Build history of the part. All positions in model axes, mm. A direction names the side the tool comes from. Round coordinates to 2 decimals unless told otherwise and drop trailing zeros. Order: outer loops, then holes, each group sorted by start corner. A loop starts at its lowest first (then second) coordinate and runs counter-clockwise, first axis right, second up. Notation, with made-up numbers: M 1,42.5 L 57,42.5 A17 ccw 57,49.5 Z; hole C 39,78 d6. An arc over 180 degrees is marked long. Use CSV: the item, a comma, the result in double quotes.
Autodesk Fusion 360 part; units mm, degrees
sketch "Sketch1" plane through (0, 0, 0) normal (0, 0, 1) x (1, 0, 0)
  line L0 (22, 1.5) -> (22, -1.5)
  line L1 (-22, -1.5) -> (-22, 1.5)
  circle A0 centre (-17.5, 0) radius 2.05
  circle A1 centre (17.5, 0) radius 2.05
  line L2 (-20, 3.5) -> (-13.5554, 3.5)
  line L3 (13.5554, 3.5) -> (20, 3.5)
  line L4 (20, -3.5) -> (13.5554, -3.5)
  line L5 (-13.5554, -3.5) -> (-20, -3.5)
  arc A2 (2.9858, -13.6779) -> (13.5554, -3.5) centre (0, 0) ccw
  arc A3 (22, 1.5) -> (20, 3.5) centre (20, 1.5) ccw
  arc A4 (20, -3.5) -> (22, -1.5) centre (20, -1.5) ccw
  arc A5 (-20, 3.5) -> (-22, 1.5) centre (-20, 1.5) ccw
  arc A6 (-22, -1.5) -> (-20, -3.5) centre (-20, -1.5) ccw
  circle A7 centre (0, 8) radius 4.55
  circle A8 centre (0, 8) radius 2.5
  spline S0 degree 5 poles (-13.5554, 3.5) (-13.4403, 3.6899) (-13.2044, 4.0607) (-12.8333, 4.5904) (-12.3036, 5.2425) (-11.5792, 5.9613) (-10.7872, 6.5756) (-9.9224, 7.0772) (-8.9826, 7.4626) (-7.9714, 7.7375) (-6.8944, 7.9106) (-5.9846, 7.9745) (-5.2769, 7.9832) (-4.794, 7.9718) (-4.5498, 7.9619) knots 0 0 0 0 0 0 0.1 0.2 0.3 0.4 0.5 0.6 0.7 0.8 0.9 1 1 1 1 1 1
  spline S1 degree 5 poles (13.5554, 3.5) (13.4982, 3.7035) (13.3727, 4.1002) (13.1508, 4.664) (12.7869, 5.3525) (12.2112, 6.1007) (11.5055, 6.7281) (10.6616, 7.2269) (9.6796, 7.5974) (8.5689, 7.8482) (7.3412, 7.9903) (6.2741, 8.0248) (5.429, 8.0092) (4.8462, 7.9807) (4.5498, 7.9619) knots 0 0 0 0 0 0 0.1 0.2 0.3 0.4 0.5 0.6 0.7 0.8 0.9 1 1 1 1 1 1
  spline S2 degree 5 poles (-13.5554, -3.5) (-13.2832, -3.5207) (-12.7507, -3.5722) (-11.9881, -3.6799) (-11.0436, -3.8844) (-9.9844, -4.2425) (-9.0464, -4.7029) (-8.2259, -5.2635) (-7.5154, -5.9188) (-6.9, -6.6582) (-6.3595, -7.4662) (-5.8692, -8.3231) (-5.4024, -9.2053) (-4.9312, -10.086) (-4.4284, -10.9351) (-3.8687, -11.7217) (-3.2294, -12.4165) (-2.4919, -12.994) (-1.6428, -13.4356) (-0.6752, -13.7313) (0.4139, -13.8766) (1.3823, -13.872) (2.163, -13.8011) (2.7075, -13.724) (2.9858, -13.6779) knots 0 0 0 0 0 0 0.05 0.1 0.15 0.2 0.25 0.3 0.35 0.4 0.45 0.5 0.55 0.6 0.65 0.7 0.75 0.8 0.85 0.9 0.95 1 1 1 1 1 1
  point P0 (-22, 3.5)
  point P1 (22, 3.5)
  point P2 (-22, -3.5)
  point P3 (-10, 7)
  point P4 (11, 7)
  point P5 (-8.024, -5.4772)
  point P6 (-5.3692, -9.2647)
  point P7 (-2.6437, -12.8398)
  dimension "d1" = 44
  dimension "d2" = 28
  dimension "d3" = 7
  dimension "d4" = 3.5
  dimension "d5" = 22
  dimension "d6" = 4.1
  dimension "d7" = 17.5
  dimension "d8" = 4.1
  dimension "d9" = 17.5
  dimension "d10" = 2
  dimension "d11" = 9.1
  dimension "d12" = 8
  dimension "d38" = 5
extrude "Extrude1" add sketch "Sketch1" along normal blind 2 contours L0 L1 L2 L3 L4 L5 A2 A3 A4 A5 A6 A7 S0 S1 S2
ref_plane "WorkPlane2" through (2.5, 0, 12.125) normal (1, 0, 0) x (0, 0, 1)
sketch "Sketch3" plane through (2.5, 0, 12.125) normal (1, 0, 0) x (0, 1, 0)
  line L0 (-4.0924, 9) -> (1.5, 9)
  line L1 (1.5, 9) -> (1.5, -11)
  line L2 (1.5, -11) -> (-11.5, -11)
  line L3 (-11.5, -11) -> (-11.5, -5.1958)
  circle A0 centre (-1.5, 7) radius 0.95
  circle A1 centre (-1.5, 0) radius 0.95
  line L4 (-4.5, -3) -> (1.5, -3)
  line L5 (1.5, -3) -> (1.5, -11)
  line L6 (1.5, -11) -> (-4.5, -11)
  line L7 (-4.5, -11) -> (-4.5, -3)
  spline S0 degree 5 poles (-10.4562, -3.7668) (-10.2158, -3.6901) (-9.7455, -3.5307) (-9.072, -3.2741) (-8.2432, -2.8843) (-7.3521, -2.2495) (-6.6362, -1.3928) (-6.1133, -0.2594) (-5.7654, 1.1445) (-5.5459, 2.7614) (-5.3974, 4.5131) (-5.29, 5.9577) (-5.1959, 7.0367) (-5.1246, 7.7503) (-5.0868, 8.1057) knots 0 0 0 0 0 0 0.1 0.2 0.3 0.4 0.5 0.6 0.7 0.8 0.9 1 1 1 1 1 1
  arc A2 (-4.0924, 9) -> (-5.0868, 8.1057) centre (-4.0924, 8) ccw
  arc A3 (-10.4562, -3.7668) -> (-11.5, -5.1958) centre (-10, -5.1958) ccw
  point P0 (-6.5, -1)
  dimension "d21" = 9
  dimension "d23" = 1.5
  dimension "d32" = 1.9
  dimension "d33" = 1.9
  dimension "d34" = 7
  dimension "d35" = 3
  dimension "d36" = 8
  dimension "d37" = 6
  dimension "d47" = 1
  dimension "d48" = 1.5
  dimension "d73" = 5.5924
  dimension "d74" = 13
  dimension "d75" = 10
  dimension "d88" = 2
  dimension "d89" = 3
extrude "Extrude12" add 1 faces at (-0.4768, -5.597, 2) along direction (0, 0, 1) blind 1
extrude "Extrude5" add sketch "Sketch3" along normal blind -1 and the other way blind -1 contours L0 L1 L2 L3 L4 L7 S0 A2 A3 | L1 L2 L4 L5 L6 L7 | A0 | A1
extrude "Extrude6" add sketch "Sketch3" along normal blind 8 contours L1 L2 L4 L5 L6 L7 | A0 | A1
fillet "Fillet1" radius 0.75 1 edges at (10.5, -2.3857, 11.7815)
fillet "Fillet2" radius 0.75 1 edges at (10.5, -2.3857, 18.7815)
fillet "Fillet4" radius 0.5 1 edges at (2.5, 1.5, 21.125)
fillet "Fillet3" radius 0.25 2 edges at (7, -4.5, 9.125) (7, 1.5, 9.125)
(1) Cut at C-C, the plane x = 6. Count the separate pieces of the cut face and the enclosed holes in it, and give its area (3 significant figures).
Answer block:
separate pieces,"3"
enclosed holes,"0"
area,"104 mm²"
(2) Two-plate mould, pull along Y, no slides. Class faces 1 (the face through (15.45, -0.09, 1.48)), 2 (the face through (2.51, -4.75, 20.88)), 3 (the face through (3, -2, 21.125)): released by +Y, released by -Y, zero draft, split by the parting line, or undercut.
Answer block:
face 1,"undercut"
face 2,"released by -Y"
face 3,"zero draft"
(3) Wall check: line 1 (Y direction, x = 17.5, z = 0.9); line 2 (Z direction, x = -2, y = 2.5); line 3 (Y direction, x = 7.5, z = 4). Give the ranges that are in metal, low to high. Write a range as from..to.
Answer block:
line 1,"y = -3.5..-2.05, 2.05..3.5"
line 2,"z = 0..3"
line 3,"y = -4.5..1.5"
(4) Cut at B-B, the plane z = 3.5. Give the cut face in (x, y), and give its area (3 significant figures).
Answer block:
outline,"M 1.5,-11.5 L 3.5,-11.5 L 3.5,-4.5 L 10.5,-4.5 L 10.5,1.5 L 1.5,1.5 Z"
area,"68.0 mm²"
(5) Cut at A-A, the plane x = 17.5. Give the cut face in (y, z).
Answer block:
outline,"M -3.5,0 L -2.05,0 L -2.05,3 L -3.5,3 Z; M 2.05,0 L 3.5,0 L 3.5,3 L 2.05,3 Z"
(6) Cut at D-D, the plane x = -17. Give the cut face in (y, z), and give its area (3 significant figures).
Answer block:
outline,"M -3.5,0 L -1.99,0 L -1.99,3 L -3.5,3 Z; M 1.99,0 L 3.5,0 L 3.5,3 L 1.99,3 Z"
area,"9.07 mm²"
(7) Tool access for faces 4 (the face through (7, -4.5, 6)), 5 (the face through (1.5, -4, 10)), 6 (the face through (3, -11.5, 5)): list every direction of +Z, -Z, +X, -X, +Y, -Y with a clear straight run to the whole face (end or side of a thin tool).
Answer block:
face 4,"+Z, +X, -Y"
face 5,"+Z, -X, +Y, -Y"
face 6,"+Z, +X, -X, -Y"
(8) Drop flat-ended pins along their axis: pin 1 (8 mm diameter, centred on x = 1, z = 14, fed in from -Y); pin 2 (4.5 mm diameter, centred on x = 8.5, z = 5.5, fed in from -Y); pin 3 (3.5 mm diameter, centred on x = 18, z = 1.5, fed in from +Y). Give the stop position or say it passes through.
Answer block:
pin 1,"stops at y = -7.29"
pin 2,"stops at y = -4.5"
pin 3,"stops at y = 3.5"
